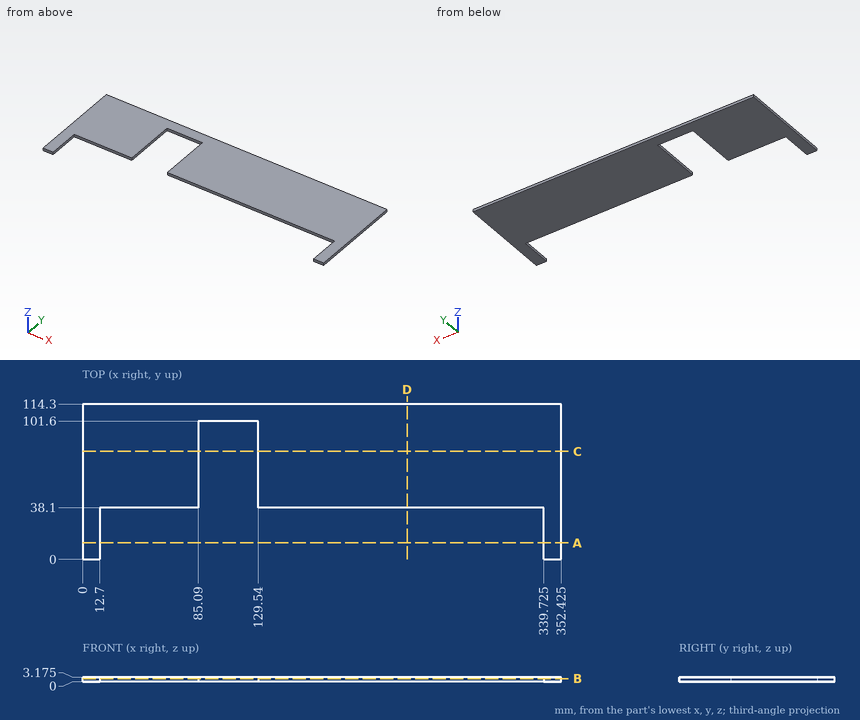
Input: dimensioned drawing with shaded views. Units: mm. Origin: part minimum x, y, z. Round coordinates to 2 decimals unless told otherwise and drop trailing zeros. Order: outer loops, then holes, each group sorted by start corner. A loop starts at its lowest first (then second) coordinate and runs counter-clockwise, first axis right, second up. Notation, with made-up numbers: (17, 6.25) -> (64, 6.25) arc R30 ccw to (64, 42.25) -> close; hole circle Ø1 at (-5, 82). An arc over 180 degrees is marked (long way). Put each result on its own line as item: value. Start each with the question number.
Q1. First-contact query: pin 1 (1.6 mm diameter, centred on x = 61.5, z = 2, fed in from -Y); pin 2 (1 mm diameter, centred on x = 107, z = 2.5, fed in from -Y). Flat tips, straight axial feed; report the tip coordinate or a pass-through.
Q2. Section C-C on y = 79.5. Return the cut outline in (x, z) (3 decimals), and give its area (3 significant figures).
Q3. Section D-D on x = 239. Return the cut outline in (y, z) (3 decimals).
Q4. Section A-A on y = 12. Return the cut outline in (x, z) (3 decimals).
Q5. Section B-B on z = 2.2. Return the cut outline in (x, y) (3 decimals).
Q6. Line query: probe 1 along X at (y, z) = (68, 2.8) (3 decimals); probe 2 along X at (y, z) = (24, 2.55) (3 decimals); probe 3 along Y at (x, z) = (73.5, 1.75). Output: solid intervals per line, ascending.
Ans:
1. pin 1: stops at y = 38.1
1. pin 2: stops at y = 101.6
2. outline: (0, 0) -> (85.09, 0) -> (85.09, 3.175) -> (0, 3.175) -> close; (129.54, 0) -> (352.425, 0) -> (352.425, 3.175) -> (129.54, 3.175) -> close
2. area: 978 mm2
3. outline: (38.1, 0) -> (114.3, 0) -> (114.3, 3.175) -> (38.1, 3.175) -> close
4. outline: (0, 0) -> (12.7, 0) -> (12.7, 3.175) -> (0, 3.175) -> close; (339.725, 0) -> (352.425, 0) -> (352.425, 3.175) -> (339.725, 3.175) -> close
5. outline: (0, 0) -> (12.7, 0) -> (12.7, 38.1) -> (85.09, 38.1) -> (85.09, 101.6) -> (129.54, 101.6) -> (129.54, 38.1) -> (339.725, 38.1) -> (339.725, 0) -> (352.425, 0) -> (352.425, 114.3) -> (0, 114.3) -> close
6. probe 1: x = 0 to 85.09, 129.54 to 352.425
6. probe 2: x = 0 to 12.7, 339.725 to 352.425
6. probe 3: y = 38.1 to 114.3
